Autodesk Fusion 360 part; units mm, degrees
sketch "Sketch1" plane through (0, 0, 0) normal (0, 1, 0) x (1, 0, 0)
  line L0 (32.5, 0) -> (27.5, -5)
  line L1 (27.5, -5) -> (32.5, -10)
  line L2 (33.4, 0) -> (28.4, -5)
  line L3 (28.4, -5) -> (33.4, -10)
  line L4 (32.5, 0) -> (33.4, 0)
  line L5 (33.4, -10) -> (32.5, -10)
  line L6 (32.5, 0) -> (0, 0) construction
  point P0 (30, -2.5)
  dimension "d1" = 0.9
  dimension "d2" = 10
  dimension "d11" = 30
  dimension "d12" = 32.5
revolve "Revolve1" add sketch "Sketch1" angle 360 about axis through (0, 0, 1.75) along (0, 0, 1) makes body 1
pattern_linear "R-Pattern1" count 6 spacing 10 along (0, 0, 1) of bodies 1 makes body 2 at (31.5756, -3.1596, 18.3333) makes body 3 at (31.5756, -3.1596, 28.3333) makes body 4 at (31.5756, -3.1596, 38.3333) makes body 5 at (31.5756, -3.1596, 48.3333) makes body 6 at (31.5756, -3.1596, 58.3333)
combine "Combine1" operation add target body 1 tool bodies 2 4 5 6 3
Geometry: final body of the model. Coordinates: model frame, mm. A direction names the side the tool comes from. Coordinates: 2 decimals unless noted, no trailing zeros. Order: outer loops, then holes, each group sorted by start corner. A loop starts at its lowest first (then second) coordinate and runs counter-clockwise, first axis right, second up. Notation, with made-up numbers: (-26.75, 44.5) -> (-4.75, 44.5) arc R30 ccw to (-4.75, 76.5) -> close; hole circle Ø11 at (73, 32). An arc over 180 degrees is marked (long way). Write each question's results on one line, items separated by ' | '. Start each with the question number.
1) Material intervals for line 1 along X through (y, z) = (-6, 6); line 2 along X through (y, z) = (-26, 37.5); line 3 along Y through (x, z) = (-23, 24.5), sorted ascending.
2) First-contact query: pin 1 (2 mm diameter, centred on x = -23.5, y = 17.5, fed in from -Z); pin 2 (8 mm diameter, centred on x = -24.5, y = -9.5, fed in from +Z); pin 3 (2 mm diameter, centred on y = 16.5, z = 9.5, fed in from +X). Flat tips, straight axial feed; report the tip coordinate or a pass-through.
3) Set-up query: faces 4 (the conical face through (26.5, -8.4, 4.7)), 5 (the conical face through (-21.163, -19.405, 54.687)). Return all of +Z, -Z, +X, -X, +Y, -Y with unobstructed straight access to the full face (end or side cutting, diameter ignored); none if empty.
4) Cut plane B-B, the plane z = 22. Output: boundary loops of the cut face in (x, y).
5) Cut plane A-A, the plane z = 44. Output: boundary loops of the cut face in (x, y).
6) Mould query, pull axis Y, two halves, no side actions, for faces 1 (the conical face through (26.5, -8.4, 14.7)), 2 (the conical face through (-6.22, -28.03, 25.31)), 3 (the flat face through (7, -32, 60)). Classes: released by +Y, released by -Y, zero draft, split by the parting line, or undercut.
Checks:
1) line 1: -28.78 to -27.86, 27.86 to 28.78 | line 2: -16.7 to -14.97, 14.97 to 16.7 | line 3: -17.5 to -15.97, 15.97 to 17.5
2) pin 1: z = 2.2 | pin 2: z = 57.78 | pin 3: x = 29.52
3) face 4: -Z | face 5: none
4) outline: circle Ø62.8 at (0, 0); hole circle Ø61 at (0, 0)
5) outline: circle Ø58.8 at (0, 0); hole circle Ø57 at (0, 0)
6) face 1: undercut | face 2: split by the parting line | face 3: zero draft
